Verification items for the finished model (mm, model axes). A direction names the side the tool comes from. Give positions to 0.01 mm unless a question says otherwise; leave off trailing zeros. Write each loop counter-clockwise with the first axis right and the second up, starting at its lowest first coordinate (ties: lowest second). Pieces come first, ordered by that corner, then holes.
Autodesk Fusion 360 part; units mm, degrees
sketch "Sketch1" plane through (0, 0, 0) normal (0, 1, 0) x (1, 0, 0)
  line L0 (0, 0) -> (170, 0)
  line L1 (170, 0) -> (170, -12)
  line L2 (170, -12) -> (0, -12)
  line L3 (0, -12) -> (0, 0)
  dimension "d1" = 170
  dimension "d2" = 12
extrude "Extrude1" add sketch "Sketch1" along normal blind 1.5
sketch "Sketch2" plane through (0, 1.5, 0) normal (0, 1, 0) x (-1, 0, 0)
  line L0 (0, 12) -> (-170, 12)
  line L1 (-170, 12) -> (-170, 0)
  line L2 (-170, 0) -> (0, 0)
  line L3 (0, 0) -> (0, 12)
  line L4 (-170, 6) -> (0, 6)
  line L5 (0, 6) -> (0, 4.5)
  line L6 (0, 4.5) -> (-170, 4.5)
  line L7 (-170, 4.5) -> (-170, 6)
  dimension "d5" = 1.5
extrude "Extrude2" add sketch "Sketch2" along normal blind 1.25 contours L1 L3 L4 L5 L6 L7
equation "d1 = 125 mm + 40 mm + 5 mm"
Item 1: Sectioned sample at C-C on z = 8.75. Record the cut outline in (x, y), then the cut area to 3 significant figures.
Answer key:
outline: (0, 0) - (170, 0) - (170, 1.5) - (0, 1.5) - close
area: 255 mm2
Item 2: Sectioned sample at A-A on x = 93.5. Record the cut outline in (y, z).
Answer key:
outline: (0, 0) - (1.5, 0) - (1.5, 4.5) - (2.75, 4.5) - (2.75, 6) - (1.5, 6) - (1.5, 12) - (0, 12) - close
Item 3: Sectioned sample at B-B on y = 2.1. Record the cut outline in (x, z), then the cut area to 3 significant figures.
Answer key:
outline: (0, 4.5) - (170, 4.5) - (170, 6) - (0, 6) - close
area: 255 mm2
Item 4: Depth check by flat-ended pin: pin 1 (2 mm diameter, centred on x = 116, z = 10, fed in from +Y). Enter the tip coordinate at first touch or a pass-through.
Answer key:
pin 1: stops at y = 1.5
Item 5: Scan lines: line 1 along Z through (x, y) = (117.5, 1.8); line 2 along Y through (x, z) = (51, 10.25). Record each from-to range of solid material in increasing order.
Answer key:
line 1: z = 4.5 to 6
line 2: y = 0 to 1.5
Item 6: Set-up check for faces 1 (the face through (84, 1.5, 9)), 2 (the face through (84, 1.5, 2)), 3 (the face through (84, 0, 6)): record each of +Z, -Z, +X, -X, +Y, -Y from which the full face is reachable in a straight line by a thin tool's end or side.
Answer key:
face 1: +Z, +X, -X, +Y
face 2: -Z, +X, -X, +Y
face 3: +Z, -Z, +X, -X, -Y
